from build123d import *

# Parameters (mm, degrees)
BOSS_EXTRUDE2_DEPTH = 2.5
BOSS_EXTRUDE3_DEPTH = 1.8
BOSS_EXTRUDE4_DEPTH = 2
SKETCH6_W           = 6
SKETCH6_H           = 6.3
SKETCH6_R           = 1.65
BOSS_EXTRUDE6_DEPTH = 3


with BuildPart() as part:
    # Sketch1 → Boss-Extrude2 (new body)
    with BuildSketch(Plane(origin=(0, 0, 0), x_dir=(1, 0, 0), z_dir=(0, 1, 0))):
        Polygon((0, 0), (0, 22.1), (21.7, 22.1), (21.7, 0), (17.2, 0), (17.2, 17.6), (4.5, 17.6), (4.5, 0), align=None)
    extrude(amount=BOSS_EXTRUDE2_DEPTH)

    # Sketch3 → Boss-Extrude3 (add)
    with BuildSketch(Plane(origin=(0, 2.5, 0), x_dir=(1, 0, 0), z_dir=(0, 1, 0))):
        Polygon((0, 0), (0, 22.1), (21.7, 22.1), (21.7, 0), (19, 0), (19, 19.5), (2.7, 19.5), (2.7, 0), align=None)
    extrude(amount=BOSS_EXTRUDE3_DEPTH)

    # Sketch4 → Boss-Extrude4 (add)
    with BuildSketch(Plane(origin=(0, 4.3, 0), x_dir=(1, 0, 0), z_dir=(0, 1, 0))):
        Polygon((0, 0), (0, 22.1), (21.7, 22.1), (21.7, 0), (17.45, 0), (17.45, 18), (4.25, 18), (4.25, 0), align=None)
    extrude(amount=BOSS_EXTRUDE4_DEPTH)

    # Sketch6 → Boss-Extrude6 (add)
    with BuildSketch(Plane.XY):
        with Locations((-3, 3.15)):
            Rectangle(SKETCH6_W, SKETCH6_H)
        with Locations((-3, 3.15)):
            Circle(SKETCH6_R, mode=Mode.SUBTRACT)
        with Locations((24.7, 3.15)):
            Rectangle(SKETCH6_W, SKETCH6_H)
        with Locations((24.7, 3.15)):
            Circle(SKETCH6_R, mode=Mode.SUBTRACT)
    extrude(amount=-BOSS_EXTRUDE6_DEPTH)


solid = part.part
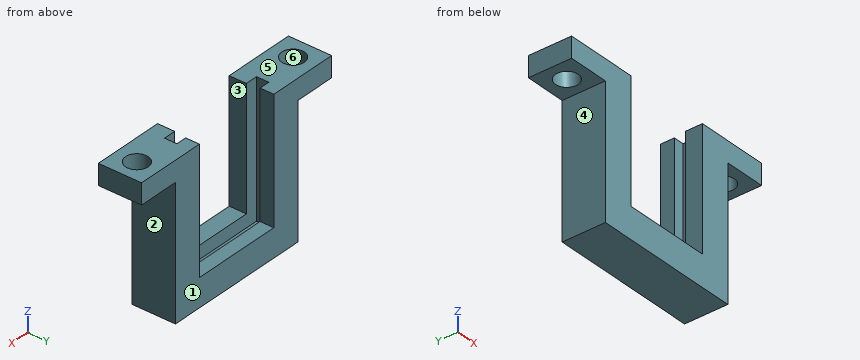
Verification items for the finished model (mm, model axes). Face numbers are marked on the shaded views. A direction names the side the tool comes from. Give positions to 0.01 mm unless a question says otherwise; leave off trailing zeros. Write each loop counter-clockwise with the first axis right and the second up, starting at its lowest first coordinate (ties: lowest second). Pieces come first, ordered by that corner, then holes. Notation, with made-up numbers: M 44,49.25 L 102,49.25 A31 ccw 102,80.25 Z; hole C -27,-28 d5. An arc over 180 degrees is marked long. Use CSV: the item, a comma, the result in double quotes.
1) Release check for a two-part mould opening along X. For the marked faces 4, 5 and 6 record: released by +X, released by -X, zero draft, split by the parting line, or undercut.
Final values:
face 4,"released by -X"
face 5,"zero draft"
face 6,"undercut"
2) Access from +Z, -Z, +X, -X, +Y, -Y to the whole of each face (thin tool, end or side, straight path). Record for the marked faces 1, 2 and 3.
Final values:
face 1,"+Z, -Z, +X, -X, +Y"
face 2,"-Z, +X, +Y, -Y"
face 3,"+Z, +Y, -Y"
3) Material ranges on line 1 along X through (y, z) = (4, -7.5); line 2 along Y through (x, z) = (24.7, -0.65); line 3 along X through (y, z) = (4.5, -1.25), recorded low to high.
Final values:
line 1,"0 to 2.7, 19 to 21.7"
line 2,"0 to 1.5, 4.8 to 6.3"
line 3,"-6 to -3.95, -2.05 to 4.25, 17.45 to 23.75, 25.65 to 27.7"
4) Cross-section at B-B (y = 3.15). Enter the section's corners in (x, z).
Final values:
outline,"M -6,-3 L -4.65,-3 L -4.65,0 L -6,0 Z; M -1.35,-3 L 0,-3 L 0,-22.1 L 21.7,-22.1 L 21.7,-3 L 23.05,-3 L 23.05,0 L 19,0 L 19,-19.5 L 2.7,-19.5 L 2.7,0 L -1.35,0 Z; M 26.35,-3 L 27.7,-3 L 27.7,0 L 26.35,0 Z"
5) Cross-section at A-A (z = -1.75). Enter the section's corners in (x, y), plus the area to 3 significant figures.
Final values:
outline,"M -6,0 L 4.5,0 L 4.5,2.5 L 2.7,2.5 L 2.7,4.3 L 4.25,4.3 L 4.25,6.3 L -6,6.3 Z; M 17.2,0 L 27.7,0 L 27.7,6.3 L 17.45,6.3 L 17.45,4.3 L 19,4.3 L 19,2.5 L 17.2,2.5 Z; hole C -3,3.15 d3.3; hole C 24.7,3.15 d3.3"
area,"108 mm²"
6) Cross-section at C-C (z = -19). Enter the section's corners in (x, y).
Final values:
outline,"M 0,0 L 21.7,0 L 21.7,6.3 L 0,6.3 Z; hole M 2.7,2.5 L 19,2.5 L 19,4.3 L 2.7,4.3 Z"
7) Go/stop test with flat-tipped pins: pin 1 Ø2 at (x, y) = (14, 5) entering from +Z; pin 2 Ø2 at (x, y) = (13.5, 1.5) entering from +Z; pin 3 Ø1.4 at (y, z) = (3, -6) entering from +X. Record where each tip stops, or that it passes through.
Final values:
pin 1,"z = -18"
pin 2,"z = -17.6"
pin 3,"x = 21.7"
8) Cross-section at D-D (x = 8.5). Enter the section's corners in (y, z), plus the area to 3 significant figures.
Final values:
outline,"M 0,-22.1 L 6.3,-22.1 L 6.3,-18 L 4.3,-18 L 4.3,-19.5 L 2.5,-19.5 L 2.5,-17.6 L 0,-17.6 Z"
area,"24.1 mm²"
